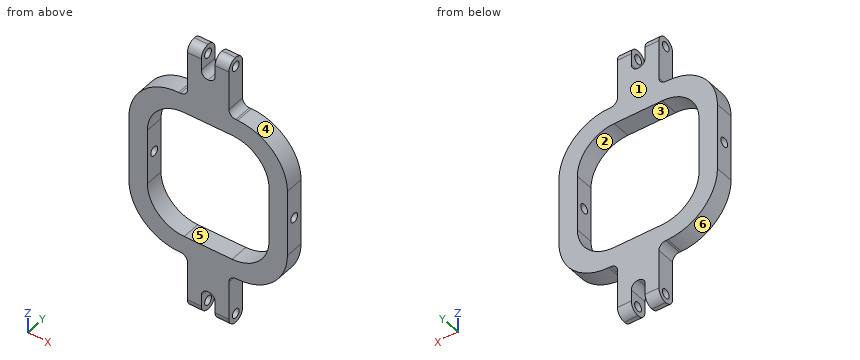
```python
from build123d import *

# Parameters (mm, degrees)
BOSS_EXTRUDE1_DEPTH      = 3.175
BOSS_EXTRUDE1_DEPTH_BACK = 3.175
SKETCH1_W                = 41.91
SKETCH1_H                = 44.704
CUT_EXTRUDE1_DEPTH       = 56.115992998
CUT_EXTRUDE1_DEPTH_BACK  = 56.115992998
SKETCH2_R                = 1.5875
FILLET1_R                = 3.175
FILLET2_R                = 12.7
FILLET4_R                = 2.38125
FILLET3_R                = 17.145


with BuildPart() as part:
    # Sketch1 → Boss-Extrude1 (new, two sides: drawn at the far end of the back side and taken through both)
    with BuildSketch(Plane(origin=(0, 0, 0), x_dir=(1, 0, 0), z_dir=(0, 1, 0)).offset(-BOSS_EXTRUDE1_DEPTH_BACK)):
        Polygon((-2.38125, -38.2466342), (2.38125, -38.2466342), (2.38125, -47.7716342), (7.14375, -47.7716342), (7.14375, -28.702), (27.305, -28.702), (27.305, 28.702), (7.14375, 28.702), (7.14375, 47.7716342), (2.38125, 47.7716342), (2.38125, 38.2466342), (-2.38125, 38.2466342), (-2.38125, 47.7716342), (-7.14375, 47.7716342), (-7.14375, 28.702), (-27.305, 28.702), (-27.305, -28.702), (-7.14375, -28.702), (-7.14375, -47.7716342), (-2.38125, -47.7716342), align=None)
        Rectangle(SKETCH1_W, SKETCH1_H, mode=Mode.SUBTRACT)
    extrude(amount=BOSS_EXTRUDE1_DEPTH + BOSS_EXTRUDE1_DEPTH_BACK)

    # Sketch2 → Cut-Extrude1 (cut, two sides: drawn at the far end of the back side and taken through both)
    with BuildSketch(Plane(origin=(0, 0, 0), x_dir=(0, 0, -1), z_dir=(1, 0, 0)).offset(-CUT_EXTRUDE1_DEPTH_BACK)):
        Circle(SKETCH2_R)
        with Locations((44.5966342, 0)):
            Circle(SKETCH2_R)
        with Locations((-44.5966342, 0)):
            Circle(SKETCH2_R)
    extrude(amount=CUT_EXTRUDE1_DEPTH + CUT_EXTRUDE1_DEPTH_BACK, mode=Mode.SUBTRACT)

    # Fillet1
    fillet1_edges = [part.edges().sort_by_distance(p)[0] for p in [
        (-4.7625, -3.175, 47.7716342),
        (-4.7625, 3.175, 47.7716342),
        (4.7625, 3.175, 47.7716342),
        (4.7625, -3.175, 47.7716342),
        (4.7625, -3.175, -47.7716342),
        (-4.7625, -3.175, -47.7716342),
        (4.7625, 3.175, -47.7716342),
        (-4.7625, 3.175, -47.7716342),
    ]]
    fillet(fillet1_edges, radius=FILLET1_R - 0.0001)  # a hair under: the kernel refuses the full size

    # Fillet2
    fillet2_edges = [part.edges().sort_by_distance(p)[0] for p in [
        (-20.955, 0, -22.352),
        (20.955, 0, -22.352),
        (20.955, 0, 22.352),
        (-20.955, 0, 22.352),
    ]]
    fillet(fillet2_edges, radius=FILLET2_R)

    # Fillet4
    fillet4_edges = [part.edges().sort_by_distance(p)[0] for p in [
        (7.14375, 0, 28.702),
        (-7.14375, 0, 28.702),
        (7.14375, 0, -28.702),
        (-7.14375, 0, -28.702),
        (-2.38125, 0, -38.2466342),
        (2.38125, 0, -38.2466342),
        (-2.38125, 0, 38.2466342),
        (2.38125, 0, 38.2466342),
    ]]
    fillet(fillet4_edges, radius=FILLET4_R - 0.0001)  # a hair under: the kernel refuses the full size

    # Fillet3
    fillet3_edges = [part.edges().sort_by_distance(p)[0] for p in [
        (-27.305, 0, 28.702),
        (-27.305, 0, -28.702),
        (27.305, 0, -28.702),
        (27.305, 0, 28.702),
    ]]
    fillet(fillet3_edges, radius=FILLET3_R)


solid = part.part
```
Source: CAD feature listing. Evaluate the final solid. Frame: model axes, mm. Face numbers are marked on the shaded views. A direction names the side the tool comes from. Give positions to 0.01 mm unless a question says otherwise; leave off trailing zeros. Loops run counter-clockwise (first coordinate to the right, second up) from the corner with the lowest first, then second, coordinate; pieces in that order, holes last. Notation, with made-up numbers: (72, -31.75) -> (101, -31.75) arc R32 cw to (101, 2.25) -> close; hole circle Ø11 at (71, 48). An arc over 180 degrees is marked (long way). Use a Markdown table: item, result. Add a question column.
(1) Section query B-B (z = 0). Output: boundary loops of the cut face in (x, y) (1 decimal).
(2) Section query C-C (x = -22). Output: boundary loops of the cut face in (y, z) (1 decimal), then the cut area to 3 significant figures.
(3) Section query A-A (x = -5). Count the separate pieces of the cut face and the enclosed holes in it, then the cut area to 3 significant figures.
(4) Ray query, line 1 (Z direction, x = -5.65, y = 0); line 2 (X direction, y = -2.25, z = 43); line 3 (X direction, y = 2, z = 0) (3 decimals). Return the intervals inside material, ascending.
(5) First-contact query: pin 1 Ø3 at (x, y) = (21, -2) entering from +Z; pin 2 Ø2 at (y, z) = (0.5, -36) entering from -X; pin 3 Ø1.5 at (y, z) = (2, 30) entering from -X. Flat tips, straight axial feed; report the tip coordinate or a pass-through.
(6) Pull-direction query (Z, two-part tool) for the marked faces 1, 2, 3 and 4; classes: +Z half, -Z half, draft (parallel to the pull), parting line (faces both ways), or undercut.
(7) Access query for the marked faces 5 and 6. Directions: +Z, -Z, +X, -X, +Y, -Y. A direction counts if a zero-diameter tool reaches every point of the face in a straight line with its end or side. Return the directions, or none.
Checked values:
| question | item | result |
|---|---|---|
| 1 | outline | (-27.3, -3.2) -> (-21, -3.2) -> (-21, -1.6) -> (-27.3, -1.6) -> close; (-27.3, 1.6) -> (-21, 1.6) -> (-21, 3.2) -> (-27.3, 3.2) -> close; (21, -3.2) -> (27.3, -3.2) -> (27.3, -1.6) -> (21, -1.6) -> close; (21, 1.6) -> (27.3, 1.6) -> (27.3, 3.2) -> (21, 3.2) -> close |
| 2 | outline | (-3.2, -24) -> (3.2, -24) -> (3.2, 24) -> (-3.2, 24) -> close; hole circle Ø3.2 at (0, 0) |
| 2 | area | 296 mm^2 |
| 3 | separate pieces | 2 |
| 3 | enclosed holes | 2 |
| 3 | area | 298 mm^2 |
| 4 | line 1 | -47.77 to -46.18, -43.01 to -22.35, 22.35 to 43.01, 46.18 to 47.77 |
| 4 | line 2 | -7.14 to -2.38, 2.38 to 7.14 |
| 4 | line 3 | -27.305 to -20.955, 20.955 to 27.305 |
| 5 | pin 1 | z = 25.93 |
| 5 | pin 2 | x = -7.14 |
| 5 | pin 3 | x = -8.01 |
| 6 | face 1 | draft |
| 6 | face 2 | undercut |
| 6 | face 3 | undercut |
| 6 | face 4 | +Z half |
| 7 | face 5 | +Y, -Y |
| 7 | face 6 | -Z, -X, +Y, -Y |
